Could you check a few things on this drawing? It's one solid part, dimensions in mm from its lowest x, y, z. Round coordinates to 2 decimals unless told otherwise and drop trailing zeros. Loops run counter-clockwise (first coordinate to the right, second up) from the corner with the lowest first, then second, coordinate; pieces in that order, holes last. Notation, with made-up numbers: (32.25, 68.5) -> (74.25, 68.5) arc R33 cw to (74.25, 102.5) -> close; hole circle Ø6 at (-27, 0). An arc over 180 degrees is marked (long way). Put each result on its own line as item: value. Start each with the question number.
1. Imagine slicing it at C-C, the plane x = 230. Please give me the cut outline in (y, z), and give its area (3 significant figures).
2. Imagine slicing it at A-A, the plane y = 47.5. Please give me the cut outline in (x, z), and give its area (3 significant figures).
3. I need wall thicknesses on line 1 (X direction, y = 82.5, z = 302.5); line 2 (X direction, y = 58, z = 267.5); line 3 (Y direction, x = 254.5, z = 78). Which ranges of each line are inside material? Lowest first, please. Write a range as [from, to].
4. If we mould it in two halves opening along X, with no side actions, what happens to the marked faces 1, 2 and 3? For each: pulls with the +X half, pulls with the -X half, needs draft (parallel to the pull), parting line crosses it, or undercut.
5. Imagine slicing it at D-D, the plane y = 117.5. Please give me the cut outline in (x, z).
6. I'm going to push flat-ended pins straight in: P1, Ø6, axis at x = 164.5, z = 187.5, coming from the +Y side; P2, Ø8, axis at x = 353.5, y = 79.5, coming from the +Z side; P3, Ø2, axis at x = 100.5, z = 381, coming from the +Y side. Where does each tip first touch, or does it pass through?
7. Imagine slicing it at B-B, the plane z = 372.5. Please give me the cut outline in (x, y), and give its area (3 significant figures).
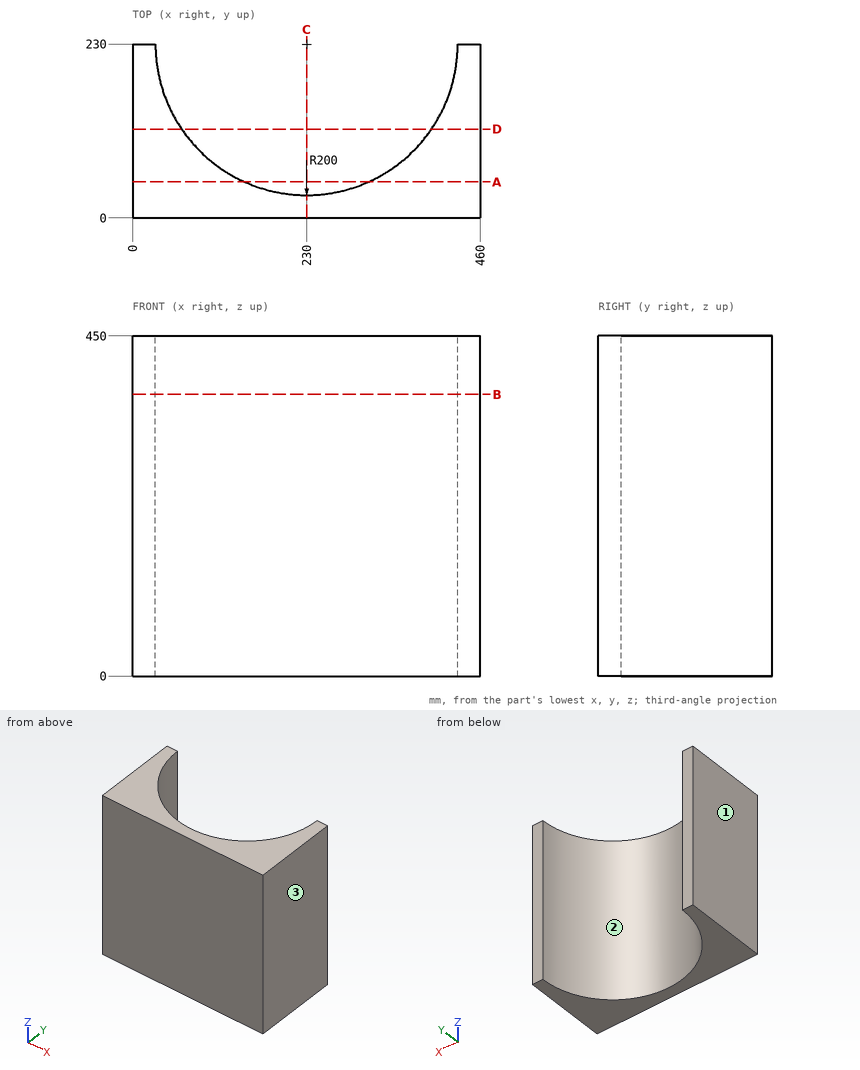
Entries:
1. outline: (0, 0) -> (30, 0) -> (30, 450) -> (0, 450) -> close
1. area: 13,500 mm^2
2. outline: (0, 0) -> (148.18, 0) -> (148.18, 450) -> (0, 450) -> close; (311.82, 0) -> (460, 0) -> (460, 450) -> (311.82, 450) -> close
2. area: 133,000 mm^2
3. line 1: [0, 94.93], [365.07, 460]
3. line 2: [0, 127.94], [332.06, 460]
3. line 3: [0, 31.51]
4. face 1: pulls with the -X half
4. face 2: undercut
4. face 3: pulls with the +X half
5. outline: (0, 0) -> (64.64, 0) -> (64.64, 450) -> (0, 450) -> close; (395.36, 0) -> (460, 0) -> (460, 450) -> (395.36, 450) -> close
6. P1: y = 42.1
6. P2: through
6. P3: y = 78.44
7. outline: (0, 0) -> (460, 0) -> (460, 230) -> (430, 230) arc R200 cw to (30, 230) -> (0, 230) -> close
7. area: 43,000 mm^2
